Check sheet for the modelled part. Datum: model origin and axes. Units: mm. A direction names the side the tool comes from. Give positions to 0.01 mm unless a question says otherwise; leave off trailing zeros. Loops run counter-clockwise (first coordinate to the right, second up) from the corner with the lowest first, then second, coordinate; pieces in that order, holes last. Notation, with made-up numbers: (39, -1.5) -> (55, -1.5) arc R26 ccw to (55, 30.5) -> close; hole circle Ø4 at (-35.5, 65.25). An arc over 180 degrees is marked (long way). Write each question's results on one line, items separated by ' | '. Start each with the question number.
Item 1: Access from +Z, -Z, +X, -X, +Y, -Y to the whole of each face (thin tool, end or side, straight path). Record for faces 1 (the face through (25.04, 6.17, -2.42)), 2 (the face through (50.8, 21, -4)), 3 (the face through (25, 25, -2.883)).
Item 2: Cross-section at B-B on z = 0. Enter the section's corners in (x, y).
Item 3: Mould release check, pull along X, two halves, no side actions. Record for faces 4 (the face through (25.044, 31.954, -2.393)), 5 (the face through (0, 21, -4)), 6 (the face through (30.948, 14.487, -4.448)): pulls with the +X half, pulls with the -X half, needs draft (parallel to the pull), parting line crosses it, or undercut.
Item 4: Cross-section at A-A on y = 19.05. Enter the section's corners in (x, z).
Item 5: Gauge pin test, flat ends, axial feed: pin 1 Ø8 at (x, y) = (19, 25) entering from +Z; pin 2 Ø4 at (y, z) = (9.5, -3) entering from -X; pin 3 Ø6 at (x, z) = (23, 4.5) entering from +Y; pin 4 Ø3 at (x, z) = (6, -3) entering from -Y. Record the tip position at first contact, or that the pin passes through.
Item 6: Scan lines: line 1 along Y through (x, z) = (24, 0); line 2 along Y through (x, z) = (40, 1.5); line 3 along Z through (x, y) = (13.5, 26.5). Record each from-to range of solid material in increasing order.
Item 7: Cross-section at C-C on x = 27.5. Enter the section's corners in (y, z), then the cut area to 3 significant figures.
from build123d import *

# Parameters (mm, degrees)
SKETCH1_R           = 4.0259
BOSS_EXTRUDE1_DEPTH = 50.8
SKETCH7_R           = 5.1435
CUT_EXTRUDE3_DEPTH  = 68.900648282


with BuildPart() as part:
    # Sketch1 → Boss-Extrude1 (new body)
    with BuildSketch(Plane(origin=(0, 0, 0), x_dir=(0, 0, -1), z_dir=(1, 0, 0))):
        with BuildLine():
            Line((2.8829, 30.951806382), (2.8829, 7.148193618))
            ThreePointArc((2.8829, 7.148193618), (2.405961877, 6.156249638), (1.333367938, 5.909338572))
            ThreePointArc((1.333367938, 5.909338572), (-4.731572785, -3.782905152), (6.0579, 0))
            Line((6.0579, 0), (6.0579, 38.1))
            ThreePointArc((6.0579, 38.1), (-4.731572785, 41.882905152), (1.333367938, 32.190661428))
            ThreePointArc((1.333367938, 32.190661428), (2.405961877, 31.943750362), (2.8829, 30.951806382))
        make_face()
        Circle(SKETCH1_R, mode=Mode.SUBTRACT)
        with Locations((0, 38.1)):
            Circle(SKETCH1_R, mode=Mode.SUBTRACT)
    extrude(amount=BOSS_EXTRUDE1_DEPTH)

    # Sketch7 → Cut-Extrude3 (cut, through all)
    with BuildSketch(Plane.XY.offset(-2.8829)):
        with Locations((28.575, 19.05)):
            Circle(SKETCH7_R)
    extrude(amount=-CUT_EXTRUDE3_DEPTH, mode=Mode.SUBTRACT)


solid = part.part
Answer sheet:
1) face 1: +X, -X | face 2: +Z, -Z, +X, +Y, -Y | face 3: +Z, +X, -X
2) outline: (0, -6.06) -> (50.8, -6.06) -> (50.8, -4.03) -> (0, -4.03) -> close; (0, 4.03) -> (50.8, 4.03) -> (50.8, 6.06) -> (0, 6.06) -> close; (0, 32.04) -> (50.8, 32.04) -> (50.8, 34.07) -> (0, 34.07) -> close; (0, 42.13) -> (50.8, 42.13) -> (50.8, 44.16) -> (0, 44.16) -> close
3) face 4: needs draft | face 5: pulls with the -X half | face 6: undercut
4) outline: (0, -6.06) -> (23.43, -6.06) -> (23.43, -2.88) -> (0, -2.88) -> close; (33.72, -6.06) -> (50.8, -6.06) -> (50.8, -2.88) -> (33.72, -2.88) -> close
5) pin 1: stops at z = -2.88 | pin 2: stops at x = 0 | pin 3: stops at y = 43.97 | pin 4: stops at y = -5.87
6) line 1: y = -6.06 to -4.03, 4.03 to 6.06, 32.04 to 34.07, 42.13 to 44.16 | line 2: y = -5.87 to -3.74, 3.74 to 5.87, 32.23 to 34.36, 41.84 to 43.97 | line 3: z = -6.06 to -2.88
7) outline: (0, -6.06) -> (14.02, -6.06) -> (14.02, -2.88) -> (7.15, -2.88) arc R1.27 cw to (5.91, -1.33) arc R6.06 ccw (long way) to start; (24.08, -6.06) -> (38.1, -6.06) arc R6.06 ccw (long way) to (32.19, -1.33) arc R1.27 cw to (30.95, -2.88) -> (24.08, -2.88) -> close; hole circle Ø8.05 at (0, 0); hole circle Ø8.05 at (38.1, 0) | area: 195 mm²
